```python
from build123d import *

# Parameters (mm, degrees)
SKETCH1_R           = 41.275
BOSS_EXTRUDE1_DEPTH = 2.54
SKETCH6_R           = 12.7
BOSS_EXTRUDE3_DEPTH = 6.35
CHAMFER2_SIZE       = 4.445
CUT_EXTRUDE2_DEPTH  = 9.89


with BuildPart() as part:
    # Sketch1 → Boss-Extrude1 (new body)
    with BuildSketch(Plane(origin=(0, 0, 0), x_dir=(1, 0, 0), z_dir=(0, 1, 0))):
        Circle(SKETCH1_R)
    extrude(amount=BOSS_EXTRUDE1_DEPTH)

    # Sketch6 → Boss-Extrude3 (add)
    with BuildSketch(Plane(origin=(0, 2.54, 0), x_dir=(1, 0, 0), z_dir=(0, 1, 0))):
        Circle(SKETCH6_R)
    extrude(amount=BOSS_EXTRUDE3_DEPTH)

    # Chamfer2
    chamfer2_edges = [part.edges().sort_by_distance(p)[0] for p in [
        (-12.7, 2.54, 0),
    ]]
    chamfer(chamfer2_edges, length=CHAMFER2_SIZE)

    # Sketch4 → Cut-Extrude2 (cut, through all)
    with BuildSketch(Plane.XZ):
        with BuildLine():
            ThreePointArc((11.86615569, 4.52596389), (9.886784934, 7.971291217), (6.939626784, 10.636333019))
            Line((6.939626784, 10.636333019), (4.098204794, 6.281299027))
            ThreePointArc((4.098204794, 6.281299027), (1.956596228, 7.240285298), (-0.376537609, 7.490541998))
            Line((-0.376537609, 7.490541998), (-0.637603684, 12.683984451))
            ThreePointArc((-0.637603684, 12.683984451), (-4.52596389, 11.86615569), (-7.971291217, 9.886784934))
            Line((-7.971291217, 9.886784934), (-4.707455443, 5.83865252))
            ThreePointArc((-4.707455443, 5.83865252), (-6.281299027, 4.098204794), (-7.240285298, 1.956596228))
            Line((-7.240285298, 1.956596228), (-12.260216438, 3.313169613))
            ThreePointArc((-12.260216438, 3.313169613), (-12.683984451, -0.637603684), (-11.86615569, -4.52596389))
            Line((-11.86615569, -4.52596389), (-7.007572258, -2.672813321))
            ThreePointArc((-7.007572258, -2.672813321), (-5.83865252, -4.707455443), (-4.098204794, -6.281299027))
            Line((-4.098204794, -6.281299027), (-6.939626784, -10.636333019))
            ThreePointArc((-6.939626784, -10.636333019), (-3.313169613, -12.260216438), (0.637603684, -12.683984451))
            Line((0.637603684, -12.683984451), (0.376537609, -7.490541998))
            ThreePointArc((0.376537609, -7.490541998), (2.672813321, -7.007572258), (4.707455443, -5.83865252))
            Line((4.707455443, -5.83865252), (7.971291217, -9.886784934))
            ThreePointArc((7.971291217, -9.886784934), (10.636333019, -6.939626784), (12.260216438, -3.313169613))
            Line((12.260216438, -3.313169613), (7.240285298, -1.956596228))
            ThreePointArc((7.240285298, -1.956596228), (7.490541998, 0.376537609), (7.007572258, 2.672813321))
            Line((7.007572258, 2.672813321), (11.86615569, 4.52596389))
        make_face()
    extrude(amount=-CUT_EXTRUDE2_DEPTH, mode=Mode.SUBTRACT)

    # Sketch7 → Revolve1 (revolve)
    with BuildSketch(Plane.XY):
        with BuildLine():
            Line((-41.275, 2.54), (-39.68496, 2.54))
            ThreePointArc((-39.68496, 2.54), (-40.47998, 3.33502), (-41.275, 2.54))
        make_face()
    revolve(axis=Axis((0, 8.001, 0), (0, -1, 0)))


solid = part.part
```
Here's how the part is built. I have some questions about the finished solid (model axes, mm). A direction names the side the tool comes from. Coordinates: 2 decimals unless noted, no trailing zeros. Order: outer loops, then holes, each group sorted by start corner. A loop starts at its lowest first (then second) coordinate and runs counter-clockwise, first axis right, second up.
1) Which directions (+Z, -Z, +X, -X, +Y, -Y) give clear straight access to the entire face, cutting with the end or side of a thin tool? Please do faces 4 (the face through (12.68, 7.92, 0.69)), 5 (the face through (-9.852, 7.924, -8.015)), 6 (the face through (17, 2.54, 8)), 7 (the face through (-4.474, 3.444, 11.886)), 8 (the face through (2, 8.89, 10)).
2) I need wall thicknesses on line 1 (X direction, y = 5, z = -9); line 2 (X direction, y = 6.5, z = -9); line 3 (Y direction, x = -31.5, z = 23). Which ranges of each line are inside material? Lowest first, please.
3) Imagine slicing it at A-A on z = 0. List the corners of the cut face in (x, y) for me (3 decimals).
4) We'd pull the mould along Z, two halves only. Please class faces 1 (the face through (-12.687, 3.444, -0.582)), 2 (the face through (-10.67, 7.92, 6.89)), 3 (the face through (-9, 8.89, 6)): +Z half, -Z half, draft (parallel to the pull), parting line (faces both ways), or undercut.
5) Will these pins go through, and if not, where does the flat tip stop? pin 1 (8 mm diameter, centred on x = 25.5, z = 7, fed in from +Y); pin 2 (3 mm diameter, centred on y = 1.5, z = 10, fed in from +X); pin 3 (2 mm diameter, centred on x = 14, z = -9, fed in from +Y).
Response values:
1. face 4: +X, +Y
1. face 5: -Z, -X, +Y
1. face 6: +Y
1. face 7: +Y, -Y
1. face 8: +Z, -Z, +X, -X, +Y
2. line 1: x = -11.6 to -5.87, 0.45 to 7.26, 8.96 to 11.6
2. line 2: x = -9.64 to -5.87, 0.45 to 7.26, 8.96 to 9.64
2. line 3: y = 0 to 2.54
3. outline: (-41.275, 0) - (-12.7, 0) - (-12.7, 6.985) - (-17.145, 2.54) - (-39.685, 2.54) arc R0.795 ccw to (-41.275, 2.54) - close; (7.5, 0) - (41.275, 0) - (41.275, 2.54) arc R0.795 ccw to (39.685, 2.54) - (17.145, 2.54) - (12.7, 6.985) - (12.7, 8.89) - (7.5, 8.89) - close
4. face 1: undercut
4. face 2: +Z half
4. face 3: draft
5. pin 1: stops at y = 2.54
5. pin 2: stops at x = 40.39
5. pin 3: stops at y = 4.04
